from build123d import *

# Parameters (mm, degrees)
SKETCH1_R                                       = 5
SKETCH1_R_2                                     = 1.6
SKETCH1_R_3                                     = 1.25
BOSS_EXTRUDE1_DEPTH                             = 3.18
CHAMFER1_SIZE                                   = 8
CHAMFER1_SIZE_2                                 = 1.410615846
CSK_FOR_M2_FLAT_HEAD_MACHINE_SCREW1_D           = 2.4
CSK_FOR_M2_FLAT_HEAD_MACHINE_SCREW1_DEPTH       = 3.508967257
CSK_FOR_M2_FLAT_HEAD_MACHINE_SCREW1_CSINK_D     = 4.4
CSK_FOR_M2_FLAT_HEAD_MACHINE_SCREW1_CSINK_ANGLE = 90
CSK_FOR_M2_FLAT_HEAD_MACHINE_SCREW1_TIP         = 0.721032743
SKETCH3_R                                       = 5
CUT_EXTRUDE4_DEPTH                              = 66.647475199
FILLET2_R                                       = 3
CHAMFER2_SIZE                                   = 1.8
FILLET4_R                                       = 0.5


# Some blends are built 0.0001 mm under size
with BuildPart() as part:
    # Sketch1 → Boss-Extrude1 (new body)
    with BuildSketch(Plane(origin=(0, 0, 0), x_dir=(0, 0, -1), z_dir=(1, 0, 0))):
        Polygon((0, 0), (0, 18.2), (-2, 20.2), (-2, 30.2), (0, 32.2), (0, 61.31), (20, 61.31), (20, 41.31), (21.8, 41.31), (21.8, 24.71), (12.6, 24.71), (12.6, 13.26), (10.25, 13.26), (10.25, 11.86), (23.25, 11.86), (23.25, 6.86), (10, 6.86), (10, 0), align=None)
        with Locations(Location((5, 25.2, 0), (0, 0, 180))):
            Circle(SKETCH1_R, mode=Mode.SUBTRACT)
        with Locations(Location((5, 56.81, 0), (0, 0, 180))):
            Circle(SKETCH1_R_2, mode=Mode.SUBTRACT)
        with Locations(Location((15, 54.81, 0), (0, 0, 180))):
            Circle(SKETCH1_R_2, mode=Mode.SUBTRACT)
        with Locations(Location((20, 9.36, 0), (0, 0, 180))):
            Circle(SKETCH1_R_3, mode=Mode.SUBTRACT)
        with Locations(Location((13.5, 9.36, 0), (0, 0, 180))):
            Circle(SKETCH1_R_3, mode=Mode.SUBTRACT)
    extrude(amount=BOSS_EXTRUDE1_DEPTH)

    # Chamfer1
    # the kernel refuses this chamfer: 8, 1.410615846 mm, written as the material it takes off along each edge
    with BuildSketch(Plane(origin=(-20.788310371, 0, -10), x_dir=(0, 0.9999776716360547, -0.006682531656101032), z_dir=(1, 0, 0))) as chamfer1_piece_1_section:
        Polygon((CHAMFER1_SIZE * 0.999977671636, CHAMFER1_SIZE * 0.0066825316561), (-CHAMFER1_SIZE_2 * 0.00668253165453, CHAMFER1_SIZE_2 * 0.999977671401), (0, 0), align=None)
    chamfer1_piece_1 = extrude(amount=44.756620743, mode=Mode.PRIVATE)
    chamfer1_piece_1 = split(chamfer1_piece_1, bisect_by=Plane(origin=(1.59, 6.86, -9.594110318), z_dir=(0, -1, 0)), keep=Keep.TOP, mode=Mode.PRIVATE)
    add(chamfer1_piece_1, mode=Mode.SUBTRACT)

    # CSK for M2 Flat Head Machine Screw1
    with Locations(Plane.ZY):
        with Locations((-4.974936087, 46.414674329), (-15.432559713, 42.244769284), (-6.592504199, 35.273154083)):
            CounterSinkHole(CSK_FOR_M2_FLAT_HEAD_MACHINE_SCREW1_D / 2, CSK_FOR_M2_FLAT_HEAD_MACHINE_SCREW1_CSINK_D / 2, depth=CSK_FOR_M2_FLAT_HEAD_MACHINE_SCREW1_DEPTH, counter_sink_angle=CSK_FOR_M2_FLAT_HEAD_MACHINE_SCREW1_CSINK_ANGLE)
            with Locations((0, 0, -(CSK_FOR_M2_FLAT_HEAD_MACHINE_SCREW1_DEPTH + CSK_FOR_M2_FLAT_HEAD_MACHINE_SCREW1_TIP / 2))):  # 118° drill point
                Cone(0, CSK_FOR_M2_FLAT_HEAD_MACHINE_SCREW1_D / 2, CSK_FOR_M2_FLAT_HEAD_MACHINE_SCREW1_TIP, mode=Mode.SUBTRACT)

    # Sketch3 → Cut-Extrude4 (cut, through all)
    with BuildSketch(Plane.ZY):
        with Locations((-9, 41.310865899)):
            Circle(SKETCH3_R)
    extrude(amount=-CUT_EXTRUDE4_DEPTH, mode=Mode.SUBTRACT)

    # Fillet2
    fillet2_edges = [part.edges().sort_by_distance(p)[0] for p in [
        (1.59, 18.2, 0),
        (1.59, 20.2, 2),
        (1.59, 30.2, 2),
        (1.59, 32.2, 0),
    ]]
    fillet(fillet2_edges, radius=FILLET2_R)

    # Chamfer2
    chamfer2_edges = [part.edges().sort_by_distance(p)[0] for p in [
        (1.59, 61.31, -20),
        (1.59, 61.31, 0),
        (1.59, 41.31, -21.8),
    ]]
    chamfer(chamfer2_edges, length=CHAMFER2_SIZE - 0.0001)  # a hair under: the kernel refuses the full size

    # Fillet4
    fillet4_edges = [part.edges().sort_by_distance(p)[0] for p in [
        (1.59, 39.5101, -21.8),
        (1.59, 59.5101, -20),
        (1.59, 59.5101, 0),
        (1.59, 0, 0),
    ]]
    fillet(fillet4_edges, radius=FILLET4_R)


solid = part.part
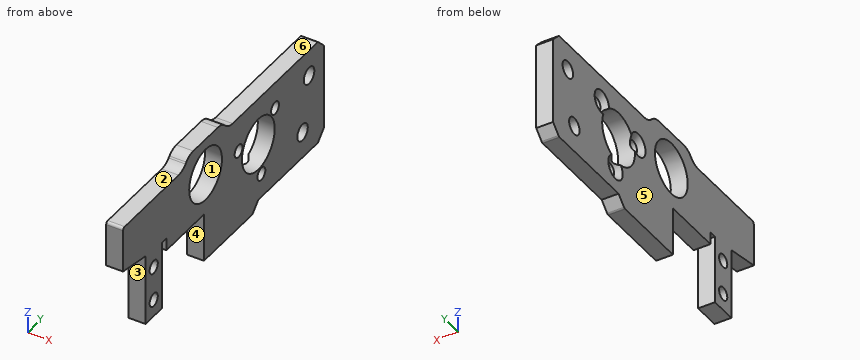
The listing builds one solid part. Answer for the finished solid, in the listing's coordinates (mm). Face numbers are marked on the shaded views. A direction names the side the tool comes from. Coordinates: 2 decimals unless noted, no trailing zeros. Write each loop counter-clockwise with the first axis right and the second up, starting at its lowest first coordinate (ties: lowest second). Pieces come first, ordered by that corner, then holes. Notation, with made-up numbers: (-18.75, 45.25) -> (22.25, 45.25) arc R29 cw to (22.25, 73.25) -> close; hole circle Ø8 at (56, -2.75). An arc over 180 degrees is marked (long way). One line per question, with ' | ' between items.
1. Which of the six approach directions +Z, -Z, +X, -X, +Y, -Y give full straight-line access (tool end or side, diameter ignored) to the marked faces 4, 5 and 6?
Verdict:
face 4: -Z, +X, -X | face 5: +Z, -Z, -X, +Y, -Y | face 6: +Z, +X, -X, +Y
2. Section B-B (y = 38.5) is taken. Determine the outline of the cut face in (x, z), and give its area (3 significant figures).
Verdict:
outline: (0, -21.8) -> (3.18, -21.8) -> (3.18, -13.14) -> (0, -13.14) -> close; (0, -4.86) -> (3.18, -4.86) -> (3.18, 0) -> (0, 0) -> close | area: 43.0 mm^2
3. Given pin 1 Ø3 at (y, z) = (35.27, -6.59) entering from -X; pin 2 Ø0.7 at (x, y) = (1, 12.5) entering from -Z; pin 3 Ø4 at (y, z) = (46.41, -4.97) entering from -X, each flat-ended and moving along its own axis, determine where each tip first touches the part or whether it passes through.
Verdict:
pin 1: stops at x = 0.7 | pin 2: stops at z = -10.25 | pin 3: stops at x = 0.19
4. Section C-C (x = 2.4) is taken. State how many separate pieces and enclosed holes the cut face has, and give its area (3 significant figures).
Verdict:
separate pieces: 1 | enclosed holes: 9 | area: 922 mm^2
5. Section D-D (y = 18) is taken. Determine the outline of the cut face in (x, z), and give its area (3 significant figures).
Verdict:
outline: (0, -12.6) -> (3.18, -12.6) -> (3.18, 0.19) -> (0, 0.19) -> close | area: 40.7 mm^2
6. Section A-A (y = 9.36) is taken. Determine the outline of the cut face in (x, z), and give its area (3 significant figures).
Verdict:
outline: (0, -23.25) -> (3.18, -23.25) -> (3.18, -21.25) -> (0, -21.25) -> close; (0, -18.75) -> (3.18, -18.75) -> (3.18, -14.75) -> (0, -14.75) -> close; (0, -12.25) -> (3.18, -12.25) -> (3.18, 0) -> (0, 0) -> close | area: 58.0 mm^2
7. For a pull along Z with two mould halves and no side action, classify the marked faces 1, 2 and 3 as released by +Z, released by -Z, zero draft, split by the parting line, or undercut.
Verdict:
face 1: undercut | face 2: released by +Z | face 3: zero draft
8. Straight lines are drawn through the part: line 1 (Z direction, x = 1.3, y = 9.36); line 2 (Y direction, x = 0.95, z = -4.75); line 3 (Z direction, x = 2.05, y = 55.5). For each, find the intervals that lie inside material, in ascending order.
Verdict:
line 1: z = -23.25 to -21.25, -18.75 to -14.75, -12.25 to 0 | line 2: y = 0 to 20.21, 30.19 to 38.68, 43.94 to 45.19, 47.64 to 55.23, 58.39 to 61.31 | line 3: z = -20 to -16.44, -13.56 to -5.92, -4.08 to 0
